Autodesk Fusion 360 part; units mm, degrees
sketch "Bottom " plane through (0, 0, 0) normal (0, 0, 1) x (1, 0, 0)
  line L0 (0, 0) -> (224, 0)
  line L1 (224, 0) -> (224, 200)
  line L2 (224, 200) -> (0, 200)
  line L3 (0, 200) -> (0, 0)
  dimension "d1" = 224
  dimension "d2" = 200
extrude "Extrude1" add sketch "Bottom " along normal blind 3
sketch "Left_Border" plane through (0, 0, 3) normal (0, 0, 1) x (-1, 0, 0)
  line L0 (0, -200) -> (0, 0)
  line L1 (0, 0) -> (-224, 0)
  line L2 (-224, 0) -> (-224, -200)
  line L3 (-224, -200) -> (0, -200)
  line L4 (0, 0) -> (-3, 0)
  line L5 (-3, 0) -> (-3, -200)
  line L6 (-3, -200) -> (0, -200)
  line L7 (0, -200) -> (0, 0)
  dimension "d5" = 3
  dimension "d6" = 200
sketch "Back_Border" plane through (0, 0, 3) normal (0, 0, 1) x (-1, 0, 0)
  line L0 (-3, -200) -> (-221, -200)
  line L1 (-221, -200) -> (-221, -197)
  line L2 (-221, -197) -> (-3, -197)
  line L3 (-3, -197) -> (-3, -200)
  dimension "d7" = 218
sketch "Right_Border" plane through (0, 0, 3) normal (0, 0, 1) x (-1, 0, 0)
  line L0 (-224, -200) -> (-221, -200)
  line L1 (-221, -200) -> (-221, 0)
  line L2 (-221, 0) -> (-224, 0)
  line L3 (-224, 0) -> (-224, -200)
  dimension "d8" = 3
  dimension "d9" = 200
extrude "Extrude2" add sketch "Left_Border" along normal blind 50 contours L0 L1 L3 L4 L5 L6 L7
extrude "Extrude3" add sketch "Back_Border" along normal blind 50
extrude "Extrude4" add sketch "Right_Border" along normal blind 50
sketch "limi_1" plane through (0, 0, 3) normal (0, 0, 1) x (-1, 0, 0)
  line L0 (-221, -197) -> (-3, -197)
  line L1 (-3, -197) -> (-3, 0)
  line L2 (-3, 0) -> (-221, 0)
  line L3 (-73, -197) -> (-73, -117)
  line L4 (-73, -197) -> (-76, -197)
  line L5 (-76, -197) -> (-76, -117)
  line L6 (-76, -117) -> (-73, -117)
  line L7 (-221, 0) -> (-221, -197)
  dimension "d17" = 80
  dimension "d18" = 3
  dimension "d19" = 80
extrude "Extrude5" add sketch "limi_1" along normal blind 50 contours L0 L3 L4 L5 L6
sketch "limi_2" plane through (0, 0, 3) normal (0, 0, 1) x (-1, 0, 0)
  line L0 (-73, -117) -> (-73, -197)
  line L1 (-73, -197) -> (-3, -197)
  line L2 (-3, -197) -> (-3, 0)
  line L3 (-3, 0) -> (-221, 0)
  line L4 (-76, -197) -> (-76, -117)
  line L5 (-76, -117) -> (-73, -117)
  line L6 (-146, -197) -> (-149, -197)
  line L7 (-149, -197) -> (-149, -117)
  line L8 (-149, -117) -> (-146, -117)
  line L9 (-146, -117) -> (-146, -197)
  line L10 (-221, 0) -> (-221, -197)
  line L11 (-221, -197) -> (-76, -197)
  dimension "d22" = 70
  dimension "d24" = 3
  dimension "d25" = 80
extrude "Extrude6" add sketch "limi_2" along normal blind 50 contours L6 L7 L8 L9 L11
sketch "Large_Front_Side" plane through (0, 0, 3) normal (0, 0, 1) x (-1, 0, 0)
  line L0 (-149, -197) -> (-149, -117)
  line L1 (-149, -117) -> (-146, -117)
  line L2 (-146, -117) -> (-146, -197)
  line L3 (-146, -197) -> (-76, -197)
  line L4 (-76, -197) -> (-76, -117)
  line L5 (-76, -117) -> (-73, -117)
  line L6 (-73, -117) -> (-73, -197)
  line L7 (-73, -197) -> (-3, -197)
  line L8 (-3, -197) -> (-3, 0)
  line L9 (-3, 0) -> (-221, 0)
  line L10 (-221, 0) -> (-221, -197)
  line L11 (-221, -197) -> (-149, -197)
  line L12 (-3, 0) -> (-73, 0)
  line L13 (-221, 0) -> (-151, 0)
  line L14 (-73, 0) -> (-151, 0)
  line L15 (-151, 0) -> (-151, -3)
  line L16 (-151, -3) -> (-73, -3)
  line L17 (-73, -3) -> (-73, 0)
  dimension "d28" = 70
  dimension "d29" = 70
  dimension "d30" = 3
extrude "Extrude7" add sketch "Large_Front_Side" along normal blind 50 contours L9 L14 L15 L16 L17
sketch "Sketch8" plane through (73, 0, 0) normal (-1, 0, 0) x (0, -1, 0)
  line L0 (-3, 3) -> (0, 3)
  line L1 (0, 3) -> (0, 53)
  line L2 (0, 53) -> (-3, 53)
  line L3 (-3, 53) -> (-3, 3)
  line L4 (-3, 53) -> (0, 53)
  line L5 (0, 53) -> (0, 43)
  line L6 (0, 43) -> (-3, 43)
  line L7 (-3, 43) -> (-3, 53)
  dimension "d33" = 3
  dimension "d34" = 10
extrude "Extrude8" add sketch "Sketch8" along normal blind 70 contours L1 L2 L3 L4 L5 L6 L7
sketch "Sketch9" plane through (151, 0, 0) normal (1, 0, 0) x (0, 1, 0)
  line L0 (0, 3) -> (3, 3)
  line L1 (3, 3) -> (3, 53)
  line L2 (3, 53) -> (0, 53)
  line L3 (0, 53) -> (0, 3)
  line L4 (0, 53) -> (3, 53)
  line L5 (3, 53) -> (3, 43)
  line L6 (3, 43) -> (0, 43)
  line L7 (0, 43) -> (0, 53)
  dimension "d37" = 3
  dimension "d38" = 10
extrude "Extrude9" add sketch "Sketch9" along normal blind 70 contours L1 L2 L3 L4 L5 L6 L7
equation "d7 = 221 mm - 3 mm"
Here's how the part is built. I have some questions about the finished solid (model axes, mm). A direction names the side the tool comes from. Round coordinates to 2 decimals unless told otherwise and drop trailing zeros. Loops run counter-clockwise (first coordinate to the right, second up) from the corner with the lowest first, then second, coordinate; pieces in that order, holes last. Notation, with made-up numbers: (70.25, 34.5) -> (112.25, 34.5) arc R19 ccw to (112.25, 41.5) -> close; hole circle Ø9 at (34.25, 1). An arc over 180 degrees is marked (long way). Answer as CSV lines item,"result". Start each with the question number.
1. Imagine slicing it at C-C on z = 49. Write out the boundary of the cut face in (x, y).
2. I need wall thicknesses on probe 1 along X at (y, z) = (132, 32.5); probe 2 along Y at (x, z) = (134.5, 36.5); probe 3 along X at (y, z) = (73, 7). Which ranges of each line are inside material? Lowest first, please. Write a range as from..to.
3. Imagine slicing it at B-B on x = 32. Write out the boundary of the cut face in (y, z).
4. Imagine slicing it at D-D on y = 30. Write out the boundary of the cut face in (x, z), plus the area to 3 significant figures.
5. If we mould it in two halves opening along Y, with no side actions, what happens to faces 1 (the face through (114, 200, 26)), 2 (the face through (73, 158, 28)), 3 (the face through (110, 0, 33))? For each: pulls with the +Y half, pulls with the -Y half, needs draft (parallel to the pull), parting line crosses it, or undercut.
6. I'm going to push flat-ended pins straight in: P1, Ø10, axis at y = 103, z = 15.5, coming from the -X side; P2, Ø6, axis at x = 71.5, y = 109, coming from the +Z side. Where does each tip first touch, or does it pass through?
7. For faces 4 (the face through (0, 101, 26)), 5 (the face through (76, 158, 28)), which set-ups out of +Z, -Z, +X, -X, +Y, -Y let a thin tool reach every point of the face, with its end or its side?
8. Imagine slicing it at A-A on z = 30.5. Write out the boundary of the cut face in (x, y).
Solution:
1,outline,"(0, 0) -> (224, 0) -> (224, 200) -> (0, 200) -> close; hole (3, 3) -> (221, 3) -> (221, 197) -> (149, 197) -> (149, 117) -> (146, 117) -> (146, 197) -> (76, 197) -> (76, 117) -> (73, 117) -> (73, 197) -> (3, 197) -> close"
2,probe 1,"0..3, 73..76, 146..149, 221..224"
2,probe 2,"0..3, 197..200"
2,probe 3,"0..3, 221..224"
3,outline,"(0, 0) -> (200, 0) -> (200, 53) -> (197, 53) -> (197, 3) -> (0, 3) -> close; (0, 43) -> (3, 43) -> (3, 53) -> (0, 53) -> close"
4,outline,"(0, 0) -> (224, 0) -> (224, 53) -> (221, 53) -> (221, 3) -> (3, 3) -> (3, 53) -> (0, 53) -> close"
4,area,"972 mm²"
5,face 1,"pulls with the +Y half"
5,face 2,"undercut"
5,face 3,"pulls with the -Y half"
6,P1,"x = 0"
6,P2,"z = 3"
7,face 4,"+Z, -Z, -X, +Y, -Y"
7,face 5,"+Z"
8,outline,"(0, 0) -> (3, 0) -> (3, 197) -> (73, 197) -> (73, 117) -> (76, 117) -> (76, 197) -> (146, 197) -> (146, 117) -> (149, 117) -> (149, 197) -> (221, 197) -> (221, 0) -> (224, 0) -> (224, 200) -> (0, 200) -> close; (73, 0) -> (151, 0) -> (151, 3) -> (73, 3) -> close"
